For this review, take the finished solid that the model builds, in its own axes (mm). A direction names the side the tool comes from. Give positions to 0.01 mm unless a question says otherwise; leave off trailing zeros. Write each loop counter-clockwise with the first axis right and the second up, starting at its lowest first coordinate (ties: lowest second). Pieces come first, ordered by that corner, then holes. Notation, with made-up numbers: (72.5, -14.5) -> (91.5, -14.5) arc R27 cw to (91.5, 1.5) -> close; hole circle Ø6 at (13, 64). An arc over 180 degrees is marked (long way). Return JSON: item names as keys, results as strings.
Autodesk Inventor part; units mm, degrees
ref_plane "YZ Plane" through (0, 0, 0) normal (1, 0, 0) x (0, 1, 0)
ref_plane "XZ Plane" through (0, 0, 0) normal (0, 1, 0) x (-1, 0, 0)
ref_plane "XY Plane" through (0, 0, 0) normal (0, 0, 1) x (1, 0, 0)
sketch "Sketch1" plane through (0, 0, 0) normal (0, 1, 0) x (-1, 0, 0)
  line L0 (0, 0) -> (60, 0)
  line L1 (60, 0) -> (60, -100)
  line L2 (60, -100) -> (0, -100)
  line L3 (0, -100) -> (0, 0)
  dimension "d0" = 100
  dimension "d1" = 60
extrude "Extrusion1" add sketch "Sketch1" along normal blind 40
sketch "Sketch2" plane through (0, 0, 0) normal (1, 0, 0) x (0, 0, -1)
  line L0 (0, 0) -> (37.6485, 44.8677)
  line L1 (0, 0) -> (58.5706, 0) construction
  line L2 (100, 40) -> (0, 40)
  line L3 (0, 40) -> (0, 0)
  point P0 (33.564, 40)
  dimension "d4" = 50
extrude "Extrusion2" cut sketch "Sketch2" against normal blind 70
sketch "Sketch3" plane through (0, 0, -100) normal (1, 0, 0) x (0, 0, -1)
  line L0 (0, 0) -> (-17, 0)
  line L1 (-100, 0) -> (0, 0)
  line L2 (0, 40) -> (-66.436, 40)
  line L3 (-17, 40) -> (-37, 40)
  line L4 (-37, 40) -> (-37, 10)
  line L5 (-37, 10) -> (-17, 10)
  line L6 (-17, 10) -> (-17, 40)
  dimension "d7" = 17
  dimension "d8" = 20
  dimension "d9" = 30
extrude "Extrusion3" add sketch "Sketch3" along normal blind 20
sketch "Sketch4" plane through (0, 10, -63) normal (0, 0, 1) x (1, 0, 0)
  line L0 (0, 30) -> (-60, 30)
  line L1 (0, 30) -> (29.4147, 5.3181)
  line L2 (0, 30) -> (38.3982, 30) construction
  line L3 (0, 30) -> (20, 30)
  line L4 (0, 30) -> (20, 30)
  line L5 (20, 30) -> (20, 13.218)
  line L6 (20, 0) -> (20, 30)
  point P0 (0, -10)
  dimension "d12" = 40
extrude "Extrusion4" cut sketch "Sketch4" against normal blind 61.75
ref_plane "Work Plane1" through (-30, 0, -100) normal (1, 0, 0) x (0, 0, -1)
mirror "Mirror1" about plane through (-30, 0, -100) normal (1, 0, 0) of "Extrusion3", "Extrusion4"
sketch "Sketch5" plane through (0, 40, -63) normal (0.6428, 0.766, 0) x (0.766, -0.6428, 0)
  circle A0 centre (12.5, 10) radius 5
  point P0 (25.7115, -63)
  dimension "d16" = 10
extrude "Extrusion5" cut sketch "Sketch5" against normal blind 27
mirror "Mirror2" about plane through (-30, 0, -100) normal (1, 0, 0) of "Extrusion5"
sketch "Sketch6" plane through (20, 10, -83) normal (0, 0, -1) x (-1, 0, 0)
  line L0 (14.2547, 25.1791) -> (31.6099, 4.4959)
  line L1 (6.5942, 18.7512) -> (23.9495, -1.932)
  line L2 (20, 30) -> (20, 18.3321)
  line L3 (20, 30) -> (20, 0)
  line L4 (20, 18.3321) -> (17, 18.3321)
  line L5 (17, 18.3321) -> (17, 27.4827)
  line L6 (17, 27.4827) -> (20, 30)
  line L7 (20, 23.9074) -> (20, 30)
  line L8 (20, 23.9074) -> (20, 30)
  point P0 (20, -10)
  dimension "d19" = 3
extrude "Extrusion6" cut sketch "Sketch6" against normal blind 81
mirror "Mirror3" about plane through (-30, 0, -100) normal (1, 0, 0) of "Extrusion6"
sketch "Sketch7" plane through (0, 0, -100) normal (0, 0, -1) x (-1, 0, 0)
  line L0 (-3, 28.3321) -> (0, 28.3321)
  line L1 (-0.0001, 31.9514) -> (2.9999, 31.9514)
  line L2 (2.9999, 31.9514) -> (2.9999, 33.9514)
  line L3 (1.4999, 33.9514) -> (2.9999, 33.9514)
  line L4 (1.4999, 33.9514) -> (1.4999, 35.4514)
  line L5 (1.4999, 35.4514) -> (2.9999, 35.4514)
  line L6 (2.9999, 35.4514) -> (2.9999, 37.4514)
  line L7 (2.9999, 37.4514) -> (-0.0001, 37.4514)
  line L8 (0, 0) -> (0, 40)
  line L9 (0, 37.4515) -> (0, 40)
  line L10 (-0.0001, 37.4514) -> (-0.0001, 31.9514)
  point P0 (0, 37.4514)
  point P1 (0, 31.9514)
  dimension "d23" = 2
  dimension "d24" = 1.5
  dimension "d25" = 2
  dimension "d26" = 1.5
  dimension "d27" = 5.5
  dimension "d28" = 3
extrude "Extrusion7" cut sketch "Sketch7" against normal blind 92.75
sketch "Sketch8" plane through (0, 0, -100) normal (0, 0, -1) x (-1, 0, 0)
  line L0 (2.9999, 37.4514) -> (0, 37.4514)
  line L1 (2.9999, 37.4514) -> (0, 37.4514)
  line L2 (0, 31.9514) -> (2.9999, 31.9514)
  line L3 (0, 37.4514) -> (0, 31.9514)
  line L4 (0, 31.9514) -> (2.9999, 31.9514)
  line L5 (2.9999, 31.9514) -> (2.9999, 33.9514)
  line L6 (2.9999, 31.9514) -> (2.9999, 33.9514)
  line L7 (2.9999, 33.9514) -> (1.4999, 33.9514)
  line L8 (1.4999, 35.4514) -> (1.4999, 33.9514)
  line L9 (1.4999, 33.9514) -> (1.4999, 35.4514)
  line L10 (1.4999, 35.4514) -> (2.9999, 35.4514)
  line L11 (2.9999, 35.4514) -> (2.9999, 37.4514)
  point P0 (0, 0)
extrude "Extrusion8" add sketch "Sketch8" against normal blind 17
sketch "Sketch9" plane through (20, 10, -83) normal (0, 0, -1) x (-1, 0, 0)
  line L0 (17, 18.3321) -> (20, 18.3321)
  line L1 (17, 18.3321) -> (17, 21.9514)
  line L2 (17, 18.3321) -> (17, 27.4827)
  line L3 (17, 21.9514) -> (15, 21.9514)
  line L4 (15, 21.9514) -> (15, 18.3321)
  line L5 (15, 18.3321) -> (17, 18.3321)
  point P0 (20, -10)
  point P1 (20, 21.9514)
  dimension "d33" = 2
  dimension "d34" = 3.6194
extrude "Extrusion9" cut sketch "Sketch9" against normal blind 69.75
mirror "Mirror4" about plane through (-30, 0, -100) normal (1, 0, 0) of "Extrusion7", "Extrusion9"
sketch "Sketch10" plane through (0, 0, -100) normal (0, 0, -1) x (-1, 0, 0)
  line L0 (60, 0) -> (60, 31.9514)
  line L1 (57.0001, 31.9514) -> (60, 31.9514)
  line L2 (60, 31.9514) -> (57.0001, 31.9514)
  line L3 (57.0001, 33.9514) -> (57.0001, 31.9514)
  line L4 (57.0001, 31.9514) -> (57.0001, 33.9514)
  line L5 (57.0001, 33.9514) -> (58.5001, 33.9514)
  line L6 (58.5001, 35.4514) -> (58.5001, 33.9514)
  line L7 (58.5001, 33.9514) -> (58.5001, 35.4514)
  line L8 (57.0001, 35.4514) -> (58.5001, 35.4514)
  line L9 (58.5001, 35.4514) -> (57.0001, 35.4514)
  line L10 (57.0001, 37.4514) -> (57.0001, 35.4514)
  line L11 (57.0001, 35.4514) -> (57.0001, 37.4514)
  line L12 (60, 37.4514) -> (57.0001, 37.4514)
  line L13 (57.0001, 37.4514) -> (60, 37.4514)
  line L14 (60, 37.4514) -> (60, 31.9514)
  point P0 (0, 0)
extrude "Extrusion10" add sketch "Sketch10" against normal blind 17
sketch "Sketch11" plane through (0, 0, -100) normal (0, 0, -1) x (-1, 0, 0)
  point P0 (0, 0)
properties part number "taslak2"
1. Add section A-A, the plane z = -47. State the section outline as (x, y) points.
Results found:
{"outline": "(-60, 0) -> (0, 0) -> (0, 31.95) -> (-3, 31.95) -> (-3, 33.95) -> (-1.5, 33.95) -> (-1.5, 35.45) -> (-3, 35.45) -> (-3, 37.45) -> (0, 37.45) -> (0, 40) -> (-60, 40) -> (-60, 37.45) -> (-57, 37.45) -> (-57, 35.45) -> (-58.5, 35.45) -> (-58.5, 33.95) -> (-57, 33.95) -> (-57, 31.95) -> (-60, 31.95) -> close"}
2. Add section C-C, the plane x = -28. State the section outline as (y, z) points, plus the area to 3 significant figures.
Results found:
{"outline": "(0, -100) -> (40, -100) -> (40, -33.56) -> (0, 0) -> close", "area": "3,330 mm²"}
3. Add section B-B, the plane y = 11.5. Count the separate pieces of the cut face and the enclosed holes in it, plus the area to 3 significant figures.
Results found:
{"separate pieces": "1", "enclosed holes": "2", "area": "6,110 mm²"}
4. The part is to be moulded in two halves that separate along Z. For faces 5 (the flat face through (-1, 31.951, -55)), 6 (the flat face through (-7.835, 11.325, -73.07)), 7 (the flat face through (10, 20, -83)), say which applies: +Z half, -Z half, draft (parallel to the pull), parting line (faces both ways), or undercut.
Results found:
{"face 5": "draft", "face 6": "undercut", "face 7": "-Z half"}
5. Add section D-D, the plane y = 4. State the section outline as (x, z) points.
Results found:
{"outline": "(-60, -100) -> (0, -100) -> (0, -3.36) -> (-60, -3.36) -> close"}
6. To check wall thickness, follow probe 1 along X at (y, z) = (34, -75); probe 2 along X at (y, z) = (11, -73); probe 3 along X at (y, z) = (10.5, -46.5). State the ranges of each line that lie inside material, in increasing order.
Results found:
{"probe 1": "x = -65.3 to -63, -58.5 to -1.5, 3 to 5.3", "probe 2": "x = -80 to -58.51, -52.55 to -7.45, -1.49 to 20", "probe 3": "x = -60 to 0"}
7. For pin 1 (6 mm diameter, centred on y = 20, z = -53.5, fed in from +X); pin 2 (16 mm diameter, centred on x = 11.5, y = 27, fed in from +Z); pin 3 (1.5 mm diameter, centred on x = -11.5, z = -18, fed in from +Y), all flat-tipped, find the tip position at first contact; note any pin that passes through.
Results found:
{"pin 1": "stops at x = 0", "pin 2": "stops at z = -63", "pin 3": "stops at y = 22.35"}
8. For faces 1 (the flat face through (5, 30, -80)), 2 (the flat face through (-70, 10, -73)), 3 (the flat face through (-70, 20, -63)), 4 (the flat face through (-63, 35, -73)), list the 3-axis set-ups (+Z, -Z, +X, -X, +Y, -Y) from which the entire face can be reached by the end or side of a thin tool; tool diameter is ignored.
Results found:
{"face 1": "+Z, -Z", "face 2": "+Z, -Z, -X, -Y", "face 3": "+Z, -X, +Y, -Y", "face 4": "+Z, -Z, +Y"}
